Can you work these out from the model? Positions are in its coordinate system, mm. A direction names the side the tool comes from. Give positions to 0.01 mm unless a question says otherwise; leave off trailing zeros. Loops run counter-clockwise (first coordinate to the right, second up) from the corner with the lowest first, then second, coordinate; pieces in that order, holes last. Notation, with made-up numbers: M 64,79 L 111,79 A32 cw 111,115 Z; hole C 89.25,-32 d6. An arc over 180 degrees is marked long. Put each result on its own line as item: value. Start each with the question number.
1) For faces 1 (the flat face through (-137, -2, -101.6)), 2 (the flat face through (-137, -80, -98.425)), 3 (the cylindrical face through (-277.628, 21.199, 6.676)), 4 (the cylindrical face through (-9.658, 21.199, 6.676)), 5 (the flat face through (-137, 81, -98.425)), which set-ups out of +Z, -Z, +X, -X, +Y, -Y let a thin tool reach every point of the face, with its end or its side?
2) Please list where these lines run through material, in increasing order: line 1 along Z through (x, y) = (-183.5, 85) (3 decimals); line 2 along Z through (x, y) = (-173, 30.5) (3 decimals); line 3 along Z through (x, y) = (-145.5, 9) (3 decimals). Write a range as from..to.
3) Imagine slicing it at D-D (x = -255). Write out the boundary of the cut face in (y, z), then the cut area to 3 significant figures.
4) Imagine slicing it at A-A (y = 0). Write out the boundary of the cut face in (x, z) (3 decimals).
5) If we mould it in two halves opening along Y, with no side actions, what happens to faces 6 (the flat face through (-137, 1, -98.425)), 7 (the flat face through (-136.979, -36.383, -88.499)), 8 (the flat face through (0, 0, -10)), 9 (the flat face through (-136.979, -39.991, -87.616))? For each: +Y half, -Y half, draft (parallel to the pull), parting line (faces both ways), or undercut.
6) For P1, Ø8, axis at x = -57.5, z = -54, coming from the +Y side; P2, Ø19.5, axis at y = -30.5, z = -88.5, coming from the +X side; P3, Ø5, axis at x = -110.5, y = 73, coming from the +Z side, each with a flat end and sliding along its axis, tell me the tip position at first contact or that it passes through.
7) Imagine slicing it at C-C (z = 0). Write out the boundary of the cut face in (x, y) (3 decimals), then the cut area to 3 significant figures.
from build123d import *

# Parameters (mm, degrees)
F2_R     = 9.525
F3_DEPTH = 69.85
F6_DEPTH = 161.925


with BuildPart() as f1:
    # F0 (on Top) → F1 (revolve)
    with BuildSketch(Plane.XY):
        Polygon((-287.02, 0), (0, 0), (0, 22.225), (-19.05, 22.225), (-22.86, 82.55), (-264.16, 82.55), (-267.97, 22.225), (-287.02, 22.225), align=None)
    revolve(axis=Axis((-143.51, 0, 0), (1, 0, 0)))

    # F2 (on face) → F3 (join)
    with BuildSketch(Plane.YZ):
        Circle(F2_R)
    extrude(amount=F3_DEPTH)

    # F5 (on offset) → F6 (join)
    with BuildSketch(Plane.YZ.offset(-57.15)):
        Polygon((-50.8, -98.425), (-109.5375, -98.425), (-109.5375, -101.6), (109.5375, -101.6), (109.5375, -98.425), (50.8, -98.425), (14.878976, -62.503976), (12.633911, -64.74904), (46.309872, -98.425), (-46.309872, -98.425), (-12.633911, -64.74904), (-14.878976, -62.503976), align=None)
    extrude(amount=-F6_DEPTH)


solid = f1.part
Recorded:
1. face 1: -Z, +X, -X, +Y, -Y
1. face 2: +X, -X, -Y
1. face 3: -X
1. face 4: +X
1. face 5: +X, -X, +Y
2. line 1: -101.6..-98.425
2. line 2: -101.6..-98.425, -82.615..-78.125, -76.709..76.709
2. line 3: -101.6..-98.425, -82.058..82.058
3. outline: C 0,0 d165.1
3. area: 21,400 mm²
4. outline: M -287.02,-22.225 L -267.97,-22.225 L -264.16,-82.55 L -22.86,-82.55 L -19.05,-22.225 L 0,-22.225 L 0,-9.525 L 69.85,-9.525 L 69.85,9.525 L 0,9.525 L 0,22.225 L -19.05,22.225 L -22.86,82.55 L -264.16,82.55 L -267.97,22.225 L -287.02,22.225 Z; M -219.075,-101.6 L -57.15,-101.6 L -57.15,-98.425 L -219.075,-98.425 Z
5. face 6: undercut
5. face 7: undercut
5. face 8: draft
5. face 9: -Y half
6. P1: y = 65.68
6. P2: x = -57.15
6. P3: z = 42.94
7. outline: M -287.02,-22.225 L -267.97,-22.225 L -264.16,-82.55 L -22.86,-82.55 L -19.05,-22.225 L 0,-22.225 L 0,-9.525 L 69.85,-9.525 L 69.85,9.525 L 0,9.525 L 0,22.225 L -19.05,22.225 L -22.86,82.55 L -264.16,82.55 L -267.97,22.225 L -287.02,22.225 Z
7. area: 43,700 mm²
